Read the model definition and answer for the solid it produces. Units are mm, in the model's axes. Face numbers are marked on the shaded views. A direction names the side the tool comes from. Coordinates: 2 decimals unless noted, no trailing zeros. Loops run counter-clockwise (first coordinate to the right, second up) from the corner with the lowest first, then second, coordinate; pieces in that order, holes last. Notation, with made-up numbers: (81, 67) - (87, 67) arc R20 cw to (87, 75) - close; hole circle Ø11 at (-4, 61.5). An arc over 180 degrees is marked (long way). Use CSV: the item, a comma, the result in double quotes.
Autodesk Fusion 360 part; units mm, degrees
sketch "Sketch1" plane through (0, 0, 0) normal (0, 1, 0) x (1, 0, 0)
  circle A0 centre (0, 0) radius 20.25
  circle A1 centre (0, 0) radius 15
  line L0 (-30, 0.6) -> (-30, -0.6)
  line L1 (30, -0.6) -> (30, 0.6)
  line L2 (30, 0.6) -> (24.8219, 2.9786)
  line L3 (24.995, -0.4999) -> (25, -0.5) construction
  line L4 (29.994, -0.5999) -> (30, -0.6) construction
  line L5 (30, 0.6) -> (29.994, 0.5999) construction
  line L6 (25, 0.5) -> (24.995, 0.4999) construction
  line L7 (25, 3) -> (25, 2.8968)
  line L8 (24.8193, -3) -> (30, -0.6)
  line L9 (25, -3) -> (24.8193, -3)
  line L10 (-25, -3) -> (-24.8219, -2.9786) construction
  line L11 (30, 0.6) -> (29.994, 0.6)
  line L12 (24.8193, 3) -> (25, 3)
  line L13 (29.994, -0.6) -> (30, -0.6)
  line L14 (14.8932, 1.7872) -> (20.1058, 2.4127) construction
  line L15 (24.8219, 2.9786) -> (25, 3) construction
  line L16 (28.7171, 8.6999) -> (28.3463, 9.8411)
  line L17 (24.5317, 4.8164) -> (28.7171, 8.6999)
  line L18 (28.3463, 9.8411) -> (22.6866, 10.5032)
  line L19 (24.6232, 17.1481) -> (23.9178, 18.119)
  line L20 (21.8426, 12.1614) -> (24.6232, 17.1481)
  line L21 (23.9178, 18.119) -> (18.3306, 16.9997)
  line L22 (18.119, 23.9178) -> (17.1481, 24.6232)
  line L23 (17.0155, 18.3159) -> (18.119, 23.9178)
  line L24 (17.1481, 24.6232) -> (12.1802, 21.8322)
  line L25 (9.8411, 28.3463) -> (8.6999, 28.7171)
  line L26 (10.5228, 22.6776) -> (9.8411, 28.3463)
  line L27 (8.6999, 28.7171) -> (4.8375, 24.5275)
  line L28 (0.6, 30) -> (-0.6, 30)
  line L29 (3, 24.8193) -> (0.6, 30)
  line L30 (-0.6, 30) -> (-2.9786, 24.8219)
  line L31 (-8.6999, 28.7171) -> (-9.8411, 28.3463)
  line L32 (-4.8164, 24.5317) -> (-8.6999, 28.7171)
  line L33 (-9.8411, 28.3463) -> (-10.5032, 22.6866)
  line L34 (-17.1481, 24.6232) -> (-18.119, 23.9178)
  line L35 (-12.1614, 21.8426) -> (-17.1481, 24.6232)
  line L36 (-18.119, 23.9178) -> (-16.9997, 18.3306)
  line L37 (-23.9178, 18.119) -> (-24.6232, 17.1481)
  line L38 (-18.3159, 17.0155) -> (-23.9178, 18.119)
  line L39 (-24.6232, 17.1481) -> (-21.8322, 12.1802)
  line L40 (-28.3463, 9.8411) -> (-28.7171, 8.6999)
  line L41 (-22.6776, 10.5228) -> (-28.3463, 9.8411)
  line L42 (-28.7171, 8.6999) -> (-24.5275, 4.8375)
  line L43 (-30, 0.6) -> (-30, -0.6)
  line L44 (-24.8193, 3) -> (-30, 0.6)
  line L45 (-30, -0.6) -> (-24.8219, -2.9786)
  line L46 (-28.7171, -8.6999) -> (-28.3463, -9.8411)
  line L47 (-24.5317, -4.8164) -> (-28.7171, -8.6999)
  line L48 (-28.3463, -9.8411) -> (-22.6866, -10.5032)
  line L49 (-24.6232, -17.1481) -> (-23.9178, -18.119)
  line L50 (-21.8426, -12.1614) -> (-24.6232, -17.1481)
  line L51 (-23.9178, -18.119) -> (-18.3306, -16.9997)
  line L52 (-18.119, -23.9178) -> (-17.1481, -24.6232)
  line L53 (-17.0155, -18.3159) -> (-18.119, -23.9178)
  line L54 (-17.1481, -24.6232) -> (-12.1802, -21.8322)
  line L55 (-9.8411, -28.3463) -> (-8.6999, -28.7171)
  line L56 (-10.5228, -22.6776) -> (-9.8411, -28.3463)
  line L57 (-8.6999, -28.7171) -> (-4.8375, -24.5275)
  line L58 (-0.6, -30) -> (0.6, -30)
  line L59 (-3, -24.8193) -> (-0.6, -30)
  line L60 (0.6, -30) -> (2.9786, -24.8219)
  line L61 (8.6999, -28.7171) -> (9.8411, -28.3463)
  line L62 (4.8164, -24.5317) -> (8.6999, -28.7171)
  line L63 (9.8411, -28.3463) -> (10.5032, -22.6866)
  line L64 (17.1481, -24.6232) -> (18.119, -23.9178)
  line L65 (12.1614, -21.8426) -> (17.1481, -24.6232)
  line L66 (18.119, -23.9178) -> (16.9997, -18.3306)
  line L67 (23.9178, -18.119) -> (24.6232, -17.1481)
  line L68 (18.3159, -17.0155) -> (23.9178, -18.119)
  line L69 (24.6232, -17.1481) -> (21.8322, -12.1802)
  line L70 (28.3463, -9.8411) -> (28.7171, -8.6999)
  line L71 (22.6776, -10.5228) -> (28.3463, -9.8411)
  line L72 (28.7171, -8.6999) -> (24.5275, -4.8375)
  arc A2 (12.1802, 21.8322) -> (10.5228, 22.6776) centre (0, 0) ccw
  arc A3 (4.8375, 24.5275) -> (3, 24.8193) centre (0, 0) ccw
  arc A4 (-2.9786, 24.8219) -> (-4.8164, 24.5317) centre (0, 0) ccw
  arc A5 (-10.5032, 22.6866) -> (-12.1614, 21.8426) centre (0, 0) ccw
  arc A6 (-16.9997, 18.3306) -> (-18.3159, 17.0155) centre (0, 0) ccw
  arc A7 (-21.8322, 12.1802) -> (-22.6776, 10.5228) centre (0, 0) ccw
  line L73 (-24.8193, -3) -> (-25, -3)
  line L74 (-24.8219, 2.9786) -> (-25, 3) construction
  line L75 (-25, 3) -> (-24.8193, 3)
  line L76 (-24.9928, 0.6) -> (-25, 0.6)
  line L77 (-25, 0.5) -> (-24.995, 0.4999) construction
  line L78 (-25, -0.6) -> (-24.9928, -0.6)
  line L79 (-24.995, -0.4999) -> (-25, -0.5) construction
  arc A8 (-24.5275, 4.8375) -> (-24.8219, 2.9786) centre (0, 0) ccw
  line L80 (-25, 2.9163) -> (-25, 3)
  line L81 (-25, -3) -> (-25, -2.8968)
  arc A9 (-24.8219, -2.9786) -> (-24.5317, -4.8164) centre (0, 0) ccw
  arc A10 (-22.6866, -10.5032) -> (-21.8426, -12.1614) centre (0, 0) ccw
  arc A11 (-18.3306, -16.9997) -> (-17.0155, -18.3159) centre (0, 0) ccw
  arc A12 (-12.1802, -21.8322) -> (-10.5228, -22.6776) centre (0, 0) ccw
  arc A13 (-4.8375, -24.5275) -> (-3, -24.8193) centre (0, 0) ccw
  arc A14 (2.9786, -24.8219) -> (4.8164, -24.5317) centre (0, 0) ccw
  arc A15 (10.5032, -22.6866) -> (12.1614, -21.8426) centre (0, 0) ccw
  arc A16 (24.5275, -4.8375) -> (24.8193, -3) centre (0, 0) ccw
  arc A17 (24.8219, 2.9786) -> (24.5317, 4.8164) centre (0, 0) ccw
  arc A18 (22.6866, 10.5032) -> (21.8426, 12.1614) centre (0, 0) ccw
  arc A19 (18.3306, 16.9997) -> (17.0155, 18.3159) centre (0, 0) ccw
  arc A20 (16.9997, -18.3306) -> (18.3159, -17.0155) centre (0, 0) ccw
  arc A21 (21.8322, -12.1802) -> (22.6776, -10.5228) centre (0, 0) ccw
  dimension "d2" = 40.5
  dimension "d3" = 30
  dimension "d4" = 50
  dimension "d5" = 50
  dimension "d6" = 6
  dimension "d7" = 60
  dimension "d8" = 1.2
  dimension "d10" = 360
extrude "Extrude1" add sketch "Sketch1" along normal blind 20 contours L0 L1 L2 L8 L16 L17 L18 L19 L20 L21 L22 L23 L24 L25 L26 L27 L28 L29 L30 L31 L32 L33 L34 L35 L36 L37 L38 L39 L40 L41 L42 L43 L44 L45 L46 L47 L48 L49 L50 L51 L52 L53 L54 L55 L56 L57 L58 L59 L60 L61 L62 L63 L64 L65 L66 L67 L68 L69 L70 L71 L72 A2 A3 A4 A5 A6 A7 A8 A9 A10 A11 A12 A13 A14 A15 A16 A17 A18 A19 A20 A21
extrude "Extrude2" add sketch "Sketch1" along normal blind 10 from surface at 5 contours A0
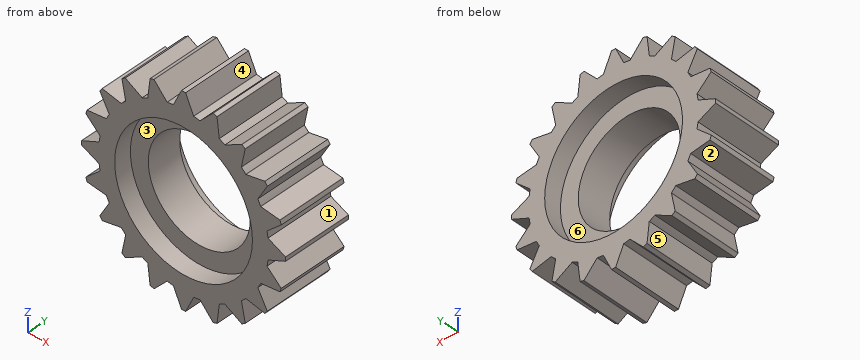
Q1. Given P1, Ø1.5, axis at x = 22, y = 18, coming from the +Z side; P2, Ø1, axis at y = 8, z = 21.5, coming from the +X side; P3, Ø1, axis at x = -7.5, y = 17, coming from the +Z side; P4, Ø12, axis at x = -7, z = -1, coming from the -Y side, each flat-ended and moving along its own axis, determine where each tip first touches the part or whether it passes through.
Reported:
P1,"stops at z = 17.89"
P2,"stops at x = 17.73"
P3,"stops at z = 27.96"
P4,"passes through"
Q2. The part is cut by section B-B on z = 7.5. Determine the outline of the cut face in (x, y).
Reported:
outline,"(-27.42, 0) - (-18.81, 0) - (-18.81, 5) - (-12.99, 5) - (-12.99, 15) - (-18.81, 15) - (-18.81, 20) - (-27.42, 20) - close; (12.99, 5) - (18.81, 5) - (18.81, 0) - (27.42, 0) - (27.42, 20) - (18.81, 20) - (18.81, 15) - (12.99, 15) - close"
Q3. Find the intervals of material crossed by probe 1 along Z at (x, y) = (0, 18.9); probe 2 along X at (y, z) = (7.25, 0), in increasing order. Write a range as [from, to].
Reported:
probe 1,"z = [-30, -20.25], [20.25, 30]"
probe 2,"x = [-30, -15], [15, 30]"
Q4. For a pull along Z with two mould halves and no side action, classify the marked faces 4, 5 and 6 as +Z half, -Z half, draft (parallel to the pull), parting line (faces both ways), or undercut.
Reported:
face 4,"+Z half"
face 5,"-Z half"
face 6,"undercut"
Q5. A tool of negligible diameter and unlimited length cuts with its end or side. For the marked faces 1, 2 and 3, from which of +Z, -Z, +X, -X, +Y, -Y can it reach the whole face along a straight path? Write none if from no direction.
Reported:
face 1,"+X, +Y, -Y"
face 2,"-X, +Y, -Y"
face 3,"-Y"
Q6. The part is cut by section A-A on x = -6.5. Determine the outline of the cut face in (y, z), and give its area (3 significant figures).
Reported:
outline,"(0, -26.35) - (20, -26.35) - (20, -19.18) - (15, -19.18) - (15, -13.52) - (5, -13.52) - (5, -19.18) - (0, -19.18) - close; (0, 19.18) - (5, 19.18) - (5, 13.52) - (15, 13.52) - (15, 19.18) - (20, 19.18) - (20, 26.33) - (0, 26.33) - close"
area,"400 mm²"
